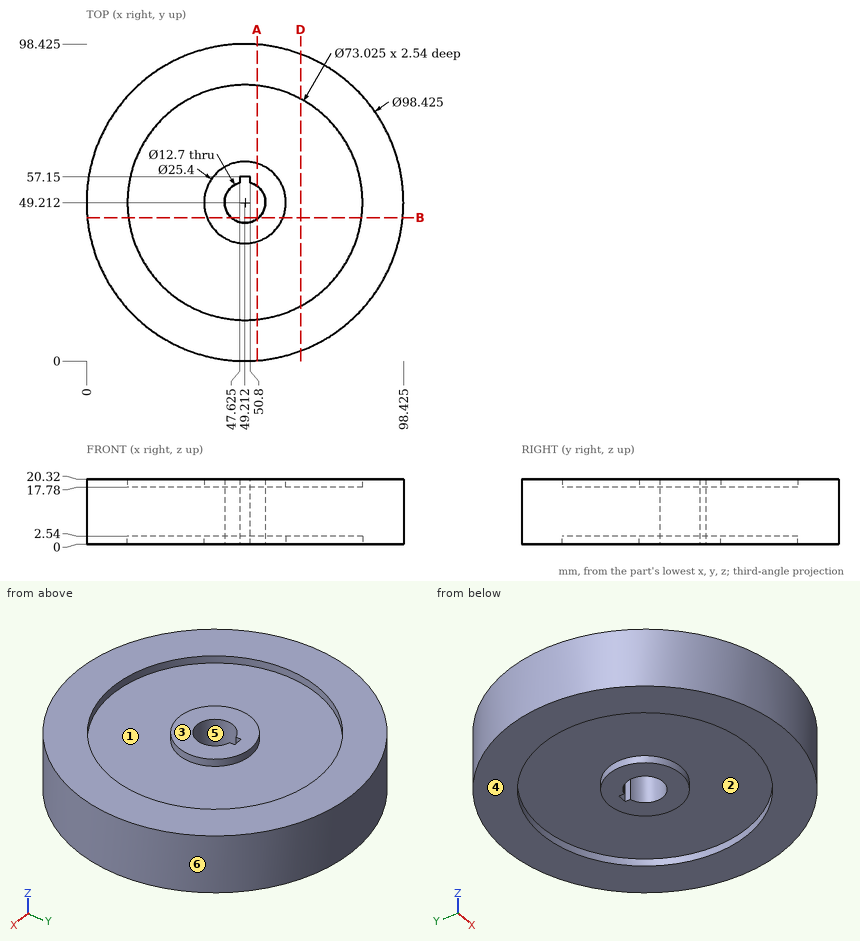
Input: dimensioned drawing with shaded views. Units: mm. Origin: part minimum x, y, z. A direction names the side the tool comes from. Coordinates: 2 decimals unless noted, no trailing zeros. Loops run counter-clockwise (first coordinate to the right, second up) from the corner with the lowest first, then second, coordinate; pieces in that order, holes last. Notation, with made-up numbers: M 16,-3 L 64,-3 A17 ccw 64,4 Z; hole C -8.75,69 d7. An arc over 180 degrees is marked long. One line per item, written item: value. Start each with the question number.
1) Cut plane B-B (y = 44.5). Return loops of the section in (x, z) (1 decimal), then the cut area to 3 significant figures.
2) Draft query along X for the marked faces 4, 5 and 6. Return one class per face: released by +X, released by -X, zero draft, split by the parting line, or undercut.
3) Cut plane A-A (x = 53). Return loops of the section in (y, z) (1 decimal).
4) Cut plane D-D (x = 66.5). Return loops of the section in (y, z), then the cut area to 3 significant figures.
5) Reachability of the marked faces 1, 2 and 3 from +Z, -Z, +X, -X, +Y, -Y: full face, straight path, thin tool, end or side. Return the list, or none.
6) Material intervals for L1, parallel to Z at x = 70.5, y = 46.5; L2, parallel to X at y = 57, z = 7 (1 decimal); L3, parallel to X at y = 48, z = 10.25 (1 decimal), sorted ascending. Write a range as from..to.
7) Pin query (flat end, axial travel): P1, Ø2, axis at x = 48, y = 30, coming from the -Z side; P2, Ø10, axis at x = 49.21, y = 49.21, coming from the +Z side; P3, Ø1.6, axis at x = 49, z = 10, coming from the -Y side; P4, Ø10, axis at x = 42.5, y = 77.5, coming from the +Z side. Return the tip coordinate at first contact, or that it passes through.
Evaluation:
1. outline: M 0.2,0 L 13,0 L 13,2.5 L 37.4,2.5 L 37.4,0 L 45,0 L 45,20.3 L 37.4,20.3 L 37.4,17.8 L 13,17.8 L 13,20.3 L 0.2,20.3 Z; M 53.5,0 L 61,0 L 61,2.5 L 85.4,2.5 L 85.4,0 L 98.2,0 L 98.2,20.3 L 85.4,20.3 L 85.4,17.8 L 61,17.8 L 61,20.3 L 53.5,20.3 Z
1. area: 1,570 mm^2
2. face 4: zero draft
2. face 5: undercut
2. face 6: split by the parting line
3. outline: M 0.1,0 L 12.9,0 L 12.9,2.5 L 37.1,2.5 L 37.1,0 L 44.1,0 L 44.1,20.3 L 37.1,20.3 L 37.1,17.8 L 12.9,17.8 L 12.9,20.3 L 0.1,20.3 Z; M 54.3,0 L 61.3,0 L 61.3,2.5 L 85.5,2.5 L 85.5,0 L 98.3,0 L 98.3,20.3 L 85.5,20.3 L 85.5,17.8 L 61.3,17.8 L 61.3,20.3 L 54.3,20.3 Z
4. outline: M 3.14,0 L 17.05,0 L 17.05,2.54 L 81.37,2.54 L 81.37,0 L 95.29,0 L 95.29,20.32 L 81.37,20.32 L 81.37,17.78 L 17.05,17.78 L 17.05,20.32 L 3.14,20.32 Z
4. area: 1,550 mm^2
5. face 1: +Z
5. face 2: -Z
5. face 3: +Z, +X, -X, +Y, -Y
6. L1: 2.54..17.78
6. L2: 0.6..47.6, 50.8..97.8
6. L3: 0..43, 55.4..98.4
7. P1: z = 2.54
7. P2: through
7. P3: y = 0
7. P4: z = 17.78
